The listing builds one solid part. Answer for the finished solid, in the listing's coordinates (mm). A direction names the side the tool comes from. Coordinates: 2 decimals unless noted, no trailing zeros. Order: outer loops, then holes, each group sorted by start corner. A loop starts at its lowest first (then second) coordinate and runs counter-clockwise, first axis right, second up. Notation, with made-up numbers: (-28, 70.5) -> (13, 70.5) arc R7 cw to (13, 80.5) -> close; hole circle Ø9 at (78.25, 2). An arc over 180 degrees is marked (long way). Return JSON: item names as keys, results as strings.
from build123d import *

# Parameters (mm, degrees)
BOSS_EXTRUDE1_DEPTH = 25
SKETCH2_R           = 6.25
CUT_EXTRUDE1_DEPTH  = 146.07239572
CUT_EXTRUDE2_START  = 2.5
CUT_EXTRUDE2_DEPTH  = 20


with BuildPart() as part:
    # Sketch1 → Boss-Extrude1 (new body)
    with BuildSketch(Plane.XY):
        with BuildLine():
            Line((-3, 75.940766391), (-3, 111))
            Line((-3, 111), (-43, 111))
            Line((-43, 111), (-43, 82.462112512))
            ThreePointArc((-43, 82.462112512), (-93, 0), (-43, -82.462112512))
            Line((-43, -82.462112512), (-43, -111))
            Line((-43, -111), (-3, -111))
            Line((-3, -111), (-3, -75.940766391))
            ThreePointArc((-3, -75.940766391), (-76, 0), (-3, 75.940766391))
        make_face()
        with BuildLine():
            Line((-3, 72.938330115), (-3, 75.940766391))
            ThreePointArc((-3, 75.940766391), (-76, 0), (-3, -75.940766391))
            Line((-3, -75.940766391), (-3, -72.938330115))
            ThreePointArc((-3, -72.938330115), (-73, 0), (-3, 72.938330115))
        make_face()
    extrude(amount=BOSS_EXTRUDE1_DEPTH)

    # Sketch2 → Cut-Extrude1 (cut, through all)
    with BuildSketch(Plane(origin=(-3, 0, 0), x_dir=(0, 0, -1), z_dir=(1, 0, 0))):
        with Locations(Location((-12.5, 95, 0), (0, 0, 90))):
            Circle(SKETCH2_R)
        with Locations(Location((-12.5, -95, 0), (0, 0, 180))):
            Circle(SKETCH2_R)
    extrude(amount=-CUT_EXTRUDE1_DEPTH, mode=Mode.SUBTRACT)

    # Sketch1_3 → Cut-Extrude2 (cut)
    with BuildSketch(Plane.XY.offset(CUT_EXTRUDE2_START)):
        with BuildLine():
            Line((-3, 72.938330115), (-3, 75.940766391))
            ThreePointArc((-3, 75.940766391), (-76, 0), (-3, -75.940766391))
            Line((-3, -75.940766391), (-3, -72.938330115))
            ThreePointArc((-3, -72.938330115), (-73, 0), (-3, 72.938330115))
        make_face()
    extrude(amount=CUT_EXTRUDE2_DEPTH, mode=Mode.SUBTRACT)


solid = part.part
1. The part is cut by section C-C on y = -95. Give the vertices of the cut face in (x, z).
Answer block:
{"outline": "(-43, 0) -> (-3, 0) -> (-3, 6.25) -> (-43, 6.25) -> close; (-43, 18.75) -> (-3, 18.75) -> (-3, 25) -> (-43, 25) -> close"}
2. The part is cut by section A-A on x = -19. Give the vertices of the cut face in (y, z), and give its area (3 significant figures).
Answer block:
{"outline": "(-111, 0) -> (-70.48, 0) -> (-70.48, 2.5) -> (-73.59, 2.5) -> (-73.59, 22.5) -> (-70.48, 22.5) -> (-70.48, 25) -> (-111, 25) -> close; (70.48, 0) -> (111, 0) -> (111, 25) -> (70.48, 25) -> (70.48, 22.5) -> (73.59, 22.5) -> (73.59, 2.5) -> (70.48, 2.5) -> close; hole circle Ø12.5 at (-95, 12.5); hole circle Ø12.5 at (95, 12.5)", "area": "1,660 mm2"}
3. For faces 1 (the face through (-75, 1, 0)), 2 (the face through (-75, 0, 2.5)), 3 (the face through (-43, -103, 12)), 4 (the face through (-43, 103, 12)), 5 (the face through (-92.99, 1.42, 12.32)), determine the directions among +Z, -Z, +X, -X, +Y, -Y from which every point of the face is accessible in a straight line to the end or side of a thin tool.
Answer block:
{"face 1": "-Z, +X, -X, +Y, -Y", "face 2": "+X", "face 3": "+Z, -Z, -X, -Y", "face 4": "+Z, -Z, -X, +Y", "face 5": "+Z, -Z, -X"}
4. The part is cut by section D-D on y = 70. Give the vertices of the cut face in (x, z).
Answer block:
{"outline": "(-61.23, 0) -> (-20.71, 0) -> (-20.71, 2.5) -> (-29.6, 2.5) -> (-29.6, 22.5) -> (-20.71, 22.5) -> (-20.71, 25) -> (-61.23, 25) -> close"}
5. Consider line 1 (Y direction, x = -17.5, z = 16); line 2 (Z direction, x = -23.5, y = -95); line 3 (Y direction, x = -66.5, z = 17). Determine where each line is inside the solid, lowest interval first. Write a range as from..to.
Answer block:
{"line 1": "y = -111..-100.18, -89.82..-73.96, 73.96..89.82, 100.18..111", "line 2": "z = 0..6.25, 18.75..25", "line 3": "y = -65.01..-36.79, 36.79..65.01"}
6. Each of these flat-tipped pins is pushed along its axis until it touches: pin 1 Ø10 at (y, z) = (-95, 12.5) entering from +X; pin 2 Ø1 at (x, z) = (-80.5, 12) entering from -Y; pin 3 Ø3 at (x, z) = (-65.5, 22) entering from +Y; pin 4 Ø12.5 at (y, z) = (-96, 18) entering from -X. Where does it stop, or does it pass through?
Answer block:
{"pin 1": "passes through", "pin 2": "stops at y = -47.42", "pin 3": "stops at y = 67.48", "pin 4": "stops at x = -43"}
7. Determine the mould class of faces 6 (the face through (-72.983, -1.563, 1.232)), 7 (the face through (-22.72, 100.773, 10.106)), 8 (the face through (-3, -88, 12)), 9 (the face through (-23, -111, 12)) for opening direction Y: pulls with the +Y half, pulls with the -Y half, needs draft (parallel to the pull), parting line crosses it, or undercut.
Answer block:
{"face 6": "undercut", "face 7": "undercut", "face 8": "needs draft", "face 9": "pulls with the -Y half"}
8. The part is cut by section B-B on z = 12.5. Give the vertices of the cut face in (x, y), and give its area (3 significant figures).
Answer block:
{"outline": "(-43, -111) -> (-3, -111) -> (-3, -101.25) -> (-43, -101.25) -> close; (-43, -88.75) -> (-3, -88.75) -> (-3, -75.94) arc R76 cw to (-3, 75.94) -> (-3, 88.75) -> (-43, 88.75) -> (-43, 82.46) arc R93 ccw to (-43, -82.46) -> close; (-43, 101.25) -> (-3, 101.25) -> (-3, 111) -> (-43, 111) -> close", "area": "5,150 mm2"}
